Design review of the part built by this model. Coordinates are the model's own, in mm. Face numbers are marked on the shaded views. A direction names the side the tool comes from. Give positions to 0.01 mm unless a question says otherwise; leave off trailing zeros. Loops run counter-clockwise (first coordinate to the right, second up) from the corner with the lowest first, then second, coordinate; pieces in that order, holes last. Notation, with made-up numbers: (48.25, 13.5) -> (86.25, 13.5) arc R11 cw to (86.25, 28.5) -> close; hole circle Ø4 at (32.25, 8). An arc over 180 degrees is marked (long way). Use a Markdown table: item, result. Add a question column.
1. Add section C-C (x = 4.25). State the section outline as (y, z) points, and give its area (3 significant figures).
2. Draft analysis for pull direction Y (two halves, no side actions). For the marked faces 1, 2 and 3, state which applies: pulls with the +Y half, pulls with the -Y half, needs draft (parallel to the pull), parting line crosses it, or undercut.
3. For pin 1 Ø1.5 at (y, z) = (-3, 2.5) entering from -X; pin 2 Ø5 at (y, z) = (-3, 11) entering from -X; pin 3 Ø1.3 at (y, z) = (0.5, 12) entering from +X, all flat-tipped, find the tip position at first contact; note any pin that passes through.
4. For the marked faces 4, 5 and 6, list the 3-axis set-ups (+Z, -Z, +X, -X, +Y, -Y) from which the entire face can be reached by the end or side of a thin tool; tool diameter is ignored.
5. Add section B-B (y = 0). State the section outline as (x, z) points.
6. To check wall thickness, follow line 1 (X direction, y = -0.25, z = 1.5); line 2 (Z direction, x = 6, y = 0); line 3 (Y direction, x = 0, z = 13.45). State the ranges of each line that lie inside material, in increasing order.
7. Add section A-A (z = 1.25). State the section outline as (x, y) points.
8. Add section D-D (z = 5.75). State the section outline as (x, y) points.
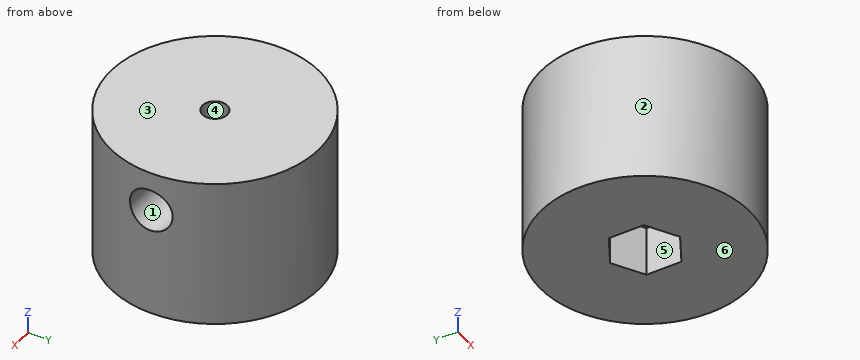
Autodesk Inventor part; units mm, degrees
ref_plane "Plano de trabajo1" through (10.5, 0, 0) normal (-1, 0, 0) x (0, 0, 1)
ref_plane "YZ Plane" through (0, 0, 0) normal (1, 0, 0) x (0, 1, 0)
ref_plane "XZ Plane" through (0, 0, 0) normal (0, 1, 0) x (-1, 0, 0)
sketch "Boceto1" plane through (0, 0, 0) normal (0, 0, 1) x (1, 0, 0)
  circle A0 centre (0, 0) radius 10.5
  dimension "d0" = 21
extrude "Extrusión1" add sketch "Boceto1" along normal blind 15
sketch "Boceto2" plane through (0, 0, 15) normal (0, 0, 1) x (1, 0, 0)
  circle A0 centre (0, 0) radius 1.25
  dimension "d3" = 2.5
extrude "Extrusión2" cut sketch "Boceto2" against normal blind 8
sketch "Boceto3" plane through (0, 0, 0) normal (0, 0, -1) x (-1, 0, 0)
  line L0 (0, 3.5218) -> (3.05, 1.7609)
  line L1 (3.05, 1.7609) -> (3.05, -1.7609)
  line L2 (3.05, -1.7609) -> (0, -3.5218)
  line L3 (0, -3.5218) -> (-3.05, -1.7609)
  line L4 (-3.05, -1.7609) -> (-3.05, 1.7609)
  line L5 (-3.05, 1.7609) -> (0, 3.5218)
  point P0 (0, 0)
  point P1 (0, 0)
  point P2 (3.05, 0)
  dimension "d6" = 6.1
extrude "Extrusión3" cut sketch "Boceto3" against normal blind 5
ref_plane "Plano de trabajo1" through (10.5, 0, 0) normal (-1, 0, 0) x (0, 0, 1)
sketch "Boceto4" plane through (10.5, 0, 0) normal (-1, 0, 0) x (0, 0, 1)
  circle A0 centre (11, 0) radius 2
  line L0 (15, -10.5) -> (15, 10.5)
  point P0 (0, 0)
  dimension "d11" = 4
  dimension "d12" = 4
hole "Agujero1" at (10.5, 0, 11) direction (-1, 0, 0) diameter 4.3 depth 12
properties part number "AcopleMotor"
Taken from the geometry:
| question | item | result |
|---|---|---|
| 1 | outline | (-9.6, 0) -> (9.6, 0) -> (9.6, 15) -> (-9.6, 15) -> close; hole circle Ø4.3 at (0, 11) |
| 1 | area | 274 mm^2 |
| 2 | face 1 | undercut |
| 2 | face 2 | parting line crosses it |
| 2 | face 3 | needs draft |
| 3 | pin 1 | stops at x = -10.26 |
| 3 | pin 2 | stops at x = -10.49 |
| 3 | pin 3 | stops at x = -1.5 |
| 4 | face 4 | +Z |
| 4 | face 5 | -Z |
| 4 | face 6 | -Z, +X, -X, +Y, -Y |
| 5 | outline | (-10.5, 0) -> (-3.05, 0) -> (-3.05, 5) -> (3.05, 5) -> (3.05, 0) -> (10.5, 0) -> (10.5, 8.85) -> (1.25, 8.85) -> (1.25, 7) -> (-1.25, 7) -> (-1.25, 8.85) -> (-1.5, 8.85) -> (-1.5, 13.15) -> (-1.25, 13.15) -> (-1.25, 15) -> (-10.5, 15) -> close; (1.25, 13.15) -> (10.5, 13.15) -> (10.5, 15) -> (1.25, 15) -> close |
| 6 | line 1 | x = -10.5 to -3.05, 3.05 to 10.5 |
| 6 | line 2 | z = 0 to 8.85, 13.15 to 15 |
| 6 | line 3 | y = -10.5 to -1.25, 1.25 to 10.5 |
| 7 | outline | circle Ø21 at (0, 0); hole (-3.05, -1.76) -> (0, -3.52) -> (3.05, -1.76) -> (3.05, 1.76) -> (0, 3.52) -> (-3.05, 1.76) -> close |
| 8 | outline | circle Ø21 at (0, 0) |
